```python
from build123d import *

# Parameters (mm, degrees)
SZKIC1_W                    = 193
SZKIC1_H                    = 192
DODANIE_WYCI_GNI_CIE1_DEPTH = 47.5
OTW_R_10_0_10_1_D           = 10
SZKIC5_R                    = 20
DODANIE_WYCI_GNI_CIE2_DEPTH = 95
ZAOKR_GLENIE1_R             = 20


with BuildPart() as part:
    # Szkic1 → Dodanie-wyci_gni_cie1 (new, symmetric)
    with BuildSketch(Plane.XY):
        Rectangle(SZKIC1_W, SZKIC1_H)
    extrude(amount=DODANIE_WYCI_GNI_CIE1_DEPTH, both=True)

    # Szkic2 → Wyci_cie-obr_t1 (revolve, cut)
    with BuildSketch(Plane(origin=(0, 0, 0), x_dir=(1, 0, 0), z_dir=(0, 1, 0)), mode=Mode.PRIVATE) as wyci_cie_obr_t1_sk:
        Polygon((-93.108465818, -10), (-93.108465818, -26.965533902), (-31.305449461, -26.965533902), (-31.305449461, -47.5), (-96.5, -47.5), (-149.784754378, -47.5), (-149.784754378, -10), align=None)
        Polygon((-93.108465818, 10), (-149.784754378, 10), (-149.784754378, 64.69075005), (-34.374339346, 64.69075005), (-34.374339346, 47.5), (-93.108465818, 31.958776917), align=None)
    revolve(wyci_cie_obr_t1_sk.sketch.rotate(Axis((0, 0, 0), (0, 0, -1)), 180), axis=Axis((0, 0, 0), (0, 0, -1)), mode=Mode.SUBTRACT)

    # Otw_r _10.0 _10_1 (through all)
    with Locations(Plane.XY.offset(10)):
        with Locations((-81.25, 81.25), (81.25, 81.25), (-81.25, -81.25)):
            Hole(OTW_R_10_0_10_1_D / 2)

    # Szkic5 → Dodanie-wyci_gni_cie2 (add)
    with BuildSketch(Plane.XZ.offset(96)):
        with Locations((76.5, 0)):
            Circle(SZKIC5_R)
    extrude(amount=-DODANIE_WYCI_GNI_CIE2_DEPTH)

    # Zaokr_glenie1
    zaokr_glenie1_edges = [part.edges().sort_by_distance(p)[0] for p in [
        (-96.5, -96, 0),
        (-96.5, 96, 0),
        (96.5, 96, 0),
    ]]
    fillet(zaokr_glenie1_edges, radius=ZAOKR_GLENIE1_R)

    # Szkic6 → Obr_t1 (revolve)
    with BuildSketch(Plane.XY, mode=Mode.PRIVATE) as obr_t1_sk:
        with BuildLine():
            Line((76.5, -96), (91.5, -96))
            Line((91.5, -96), (91.5, -102))
            Line((91.5, -102), (81.295831523, -102))
            ThreePointArc((81.295831523, -102), (88.377677323, -114.709029376), (78, -124.9058809))
            Line((78, -124.9058809), (78, -864.813984477))
            Line((78, -864.813984477), (76.5, -864.813984477))
            Line((76.5, -864.813984477), (76.5, -96))
        make_face()
    revolve(obr_t1_sk.sketch.rotate(Axis((76.5, -95.828898057, 0), (0, -1, 0)), 90), axis=Axis((76.5, -95.828898057, 0), (0, -1, 0)))


solid = part.part
```
Part model, mm, in its own coordinate system. A direction names the side the tool comes from. Give positions to 0.01 mm unless a question says otherwise; leave off trailing zeros. Loops run counter-clockwise (first coordinate to the right, second up) from the corner with the lowest first, then second, coordinate; pieces in that order, holes last. Notation, with made-up numbers: M -31.75,65 L -27.75,65 A25 cw -27.75,81 Z; hole C 5,42 d3. An arc over 180 degrees is marked long. Return JSON: item names as keys, results as strings.
1) Saw through at A-A, the plane x = 0. List the corners of the cut face in (y, z), then the cut area to 3 significant figures.
Calculated:
{"outline": "M -96,-10 L -93.11,-10 L -93.11,-31.96 L -34.37,-47.5 L 34.37,-47.5 L 93.11,-31.96 L 93.11,-10 L 96,-10 L 96,10 L 93.11,10 L 93.11,26.97 L 31.31,26.97 L 31.31,47.5 L -31.31,47.5 L -31.31,26.97 L -93.11,26.97 L -93.11,10 L -96,10 Z", "area": "14,400 mm2"}
2) Saw through at B-B, the plane y = -151.5. List the corners of the cut face in (x, z).
Calculated:
{"outline": "C 76.5,0 d3"}
3) Drill centre lines: line 1 (X direction, y = 81, z = 5); line 2 (Y direction, x = -81.25, z = -2); line 3 (X direction, y = -81, z = -3). Where is each one in solid material? Low to high.
Calculated:
{"line 1": "x = -95.86 to -86.24, -76.26 to 76.26, 86.24 to 95.86", "line 2": "y = -95.43 to -86.25, -76.25 to 76.25, 86.25 to 95.43", "line 3": "x = -95.86 to -86.24, -76.26 to 96.5"}
4) 3-axis set-ups, long thin cutter, end or side, ignore diameter. For faces 1 (the face through (29.86, -9.4, 37.38)), 2 (the face through (-90.486, -90.297, 0.14)), 3 (the face through (73, -102, -4)), 4 (the face through (91.143, -99.042, -3.252)): which of +Z, -Z, +X, -X, +Y, -Y reach the whole face in a straight line?
Calculated:
{"face 1": "+Z", "face 2": "+Z, -Z, -X, -Y", "face 3": "none", "face 4": "-Y"}
5) Flat gauge pins, fed straight in: pin 1 Ø16 at (x, y) = (-81.25, -81.25) entering from -Z; pin 2 Ø10 at (x, z) = (25, 36.5) entering from +Y; pin 3 Ø3 at (x, y) = (-2, -45) entering from +Z. Where does each tip first touch, or does it go through?
Calculated:
{"pin 1": "stops at z = -10", "pin 2": "stops at y = 24.08", "pin 3": "stops at z = 26.97"}
